Source: CAD feature listing. Evaluate the final solid. Frame: model axes, mm. Coordinates: 2 decimals unless noted, no trailing zeros. Write each loop counter-clockwise with the first axis right and the second up, starting at its lowest first coordinate (ties: lowest second). Pieces come first, ordered by that corner, then holes. Notation, with made-up numbers: (-25.75, 74.25) - (5.25, 74.25) arc R14 ccw to (5.25, 100.25) - close; hole circle Ø11 at (83, -40). An arc over 180 degrees is marked (long way). One line per question, with ' | ' between items.
from build123d import *

# Parameters (mm, degrees)
SKETCH4_R           = 2.5
SKETCH4_R_2         = 1.5
BOSS_EXTRUDE1_DEPTH = 4
SKETCH5_R           = 2.159
SKETCH5_R_2         = 3
CUT_EXTRUDE1_DEPTH  = 4
FILLET1_R           = 2.54


with BuildPart() as part:
    # Sketch4 → Boss-Extrude1 (new body)
    with BuildSketch(Plane.XY):
        Polygon((-52.467947032, -38.099537239), (-52.467947032, -112.867947032), (52.467947032, -112.867947032), (52.467947032, -38.099537239), (17.557897552, 21.15), (-17.557897552, 21.15), align=None)
        with Locations((-45.283742135, -45.283742135)):
            Circle(SKETCH4_R, mode=Mode.SUBTRACT)
        with Locations((45.283742135, -45.283742135)):
            Circle(SKETCH4_R, mode=Mode.SUBTRACT)
        with Locations((45.283742135, -105.683742135)):
            Circle(SKETCH4_R, mode=Mode.SUBTRACT)
        with Locations((-45.283742135, -105.683742135)):
            Circle(SKETCH4_R, mode=Mode.SUBTRACT)
        with Locations((-15.5, -15.5)):
            Circle(SKETCH4_R_2, mode=Mode.SUBTRACT)
        with Locations((-15.5, 15.5)):
            Circle(SKETCH4_R_2, mode=Mode.SUBTRACT)
        with Locations((15.5, 15.5)):
            Circle(SKETCH4_R_2, mode=Mode.SUBTRACT)
        with Locations((15.5, -15.5)):
            Circle(SKETCH4_R_2, mode=Mode.SUBTRACT)
        Circle(SKETCH4_R, mode=Mode.SUBTRACT)
    extrude(amount=BOSS_EXTRUDE1_DEPTH)

    # Sketch5 → Cut-Extrude1 (cut)
    with BuildSketch(Plane.XY.offset(4)):
        with Locations((0, -54.767742135)):
            Circle(SKETCH5_R)
        with Locations((0, -74.833742135)):
            Circle(SKETCH5_R)
        with Locations((0, -30.767742135)):
            Circle(SKETCH5_R_2)
        with Locations((0, -98.833742135)):
            Circle(SKETCH5_R_2)
    extrude(amount=-CUT_EXTRUDE1_DEPTH, mode=Mode.SUBTRACT)

    # Fillet1
    fillet1_edges = [part.edges().sort_by_distance(p)[0] for p in [
        (-52.467947032, -38.099537239, 2),
        (-17.557897552, 21.15, 2),
        (17.557897552, 21.15, 2),
        (52.467947032, -38.099537239, 2),
        (52.467947032, -112.867947032, 2),
        (-52.467947032, -112.867947032, 2),
    ]]
    fillet(fillet1_edges, radius=FILLET1_R)


solid = part.part
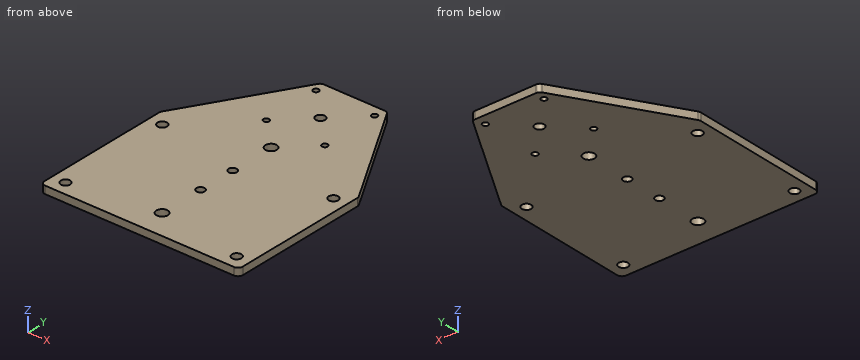
Item 1: Cut plane A-A on y = -15.5. Return loops of the section in (x, z), and give its area (3 significant figures).
Check sheet entries:
outline: (-39.15, 0) - (-17, 0) - (-17, 4) - (-39.15, 4) - close; (-14, 0) - (14, 0) - (14, 4) - (-14, 4) - close; (17, 0) - (39.15, 0) - (39.15, 4) - (17, 4) - close | area: 289 mm²
Item 2: Ray query, line 1 along Y through (x, z) = (0, 1.4); line 2 along Y through (x, z) = (15.5, 1.05); line 3 along Y through (x, z) = (47.5, 3.3). Return the intervals inside material, ascending. Write a range as [from, to].
Check sheet entries:
line 1: [-112.87, -101.83], [-95.83, -76.99], [-72.67, -56.93], [-52.61, -33.77], [-27.77, -2.5], [2.5, 21.15] | line 2: [-112.87, -17], [-14, 14], [17, 21.15] | line 3: [-112.87, -106.84], [-104.53, -46.44], [-44.13, -29.67]
Item 3: Cut plane D-D on z = 1.25. State how many separate pieces and enclosed holes the cut face has, and give its area (3 significant figures).
Check sheet entries:
separate pieces: 1 | enclosed holes: 13 | area: 11,800 mm²
Item 4: Pin query (flat end, axial travel): pin 1 Ø2 at (y, z) = (-35.5, 2) entering from +X; pin 2 Ø5 at (x, y) = (0, -54.77) entering from -Z; pin 3 Ø1.5 at (y, z) = (-16, 0.5) entering from -X; pin 4 Ø1.8 at (x, y) = (15.5, -15.5) entering from +Z. Return the tip coordinate at first contact, or that it passes through.
Check sheet entries:
pin 1: x = 51.53 | pin 2: z = 0 | pin 3: x = -39.89 | pin 4: through
Item 5: Cut plane B-B on x = 0. Return loops of the section in (y, z).
Check sheet entries:
outline: (-112.87, 0) - (-101.83, 0) - (-101.83, 4) - (-112.87, 4) - close; (-95.83, 0) - (-76.99, 0) - (-76.99, 4) - (-95.83, 4) - close; (-72.67, 0) - (-56.93, 0) - (-56.93, 4) - (-72.67, 4) - close; (-52.61, 0) - (-33.77, 0) - (-33.77, 4) - (-52.61, 4) - close; (-27.77, 0) - (-2.5, 0) - (-2.5, 4) - (-27.77, 4) - close; (2.5, 0) - (21.15, 0) - (21.15, 4) - (2.5, 4) - close
Item 6: Cut plane C-C on y = 0. Return loops of the section in (x, z), and give its area (3 significant figures).
Check sheet entries:
outline: (-30.02, 0) - (-2.5, 0) - (-2.5, 4) - (-30.02, 4) - close; (2.5, 0) - (30.02, 0) - (30.02, 4) - (2.5, 4) - close | area: 220 mm²
